Design review of the part built by this model. Coordinates are the model's own, in mm. A direction names the side the tool comes from. Coordinates: 2 decimals unless noted, no trailing zeros. Loops run counter-clockwise (first coordinate to the right, second up) from the corner with the lowest first, then second, coordinate; pieces in that order, holes last. Notation, with made-up numbers: M -2.5,56 L 27.5,56 A32 cw 27.5,89 Z; hole C -35.75,58.25 d4. An arc over 180 degrees is marked long. Answer as CSV lines item,"result". Start each with the question number.
from build123d import *

# Parameters (mm, degrees)
ESQUISSE1_W             = 55
ESQUISSE1_H             = 20
BOSS_EXTRU_1_DEPTH      = 10
ESQUISSE2_R             = 2
ENL_V_MAT_EXTRU_1_DEPTH = 20
ESQUISSE3_R             = 1.5
ESQUISSE3_W             = 23
ESQUISSE3_H             = 13
ENL_V_MAT_EXTRU_2_DEPTH = 20
BOSS_EXTRU_2_DEPTH      = 15
ENL_V_MAT_EXTRU_3_DEPTH = 15
ESQUISSE7_W             = 35
ESQUISSE7_H             = 20
ENL_V_MAT_EXTRU_4_DEPTH = 5


with BuildPart() as part:
    # Esquisse1 → Boss.-Extru.1 (new body)
    with BuildSketch(Plane.XY):
        with Locations((-0.833333333, -1.666666667)):
            Rectangle(ESQUISSE1_W, ESQUISSE1_H)
    extrude(amount=BOSS_EXTRU_1_DEPTH)

    # Esquisse2 → Enlèv. mat.-Extru.1 (cut)
    with BuildSketch(Plane(origin=(0, 8.333333333, 0), x_dir=(1, 0, 0), z_dir=(0, 1, 0))):
        with Locations(Location((-23.333333333, -5.548124667, 0), (0, 0, 270))):
            Circle(ESQUISSE2_R)
        with Locations(Location((-13.333333333, -5.548124667, 0), (0, 0, 270))):
            Circle(ESQUISSE2_R)
    extrude(amount=-ENL_V_MAT_EXTRU_1_DEPTH, mode=Mode.SUBTRACT)

    # Esquisse3 → Enlèv. mat.-Extru.2 (cut)
    with BuildSketch(Plane.XY.offset(10)):
        with Locations((24.166666667, -1.666666667)):
            Circle(ESQUISSE3_R)
        with Locations((-3.833333333, -1.666666667)):
            Circle(ESQUISSE3_R)
        with Locations((10.166666667, -1.666666667)):
            Rectangle(ESQUISSE3_W, ESQUISSE3_H)
    extrude(amount=-ENL_V_MAT_EXTRU_2_DEPTH, mode=Mode.SUBTRACT)

    # Esquisse5 → Boss.-Extru.2 (add)
    with BuildSketch(Plane(origin=(0, 0, 0), x_dir=(-1, 0, 0), z_dir=(0, 0, -1))):
        Polygon((28.333333333, -11.666666667), (28.333333333, 8.333333333), (8.333333333, 8.333333333), (8.333333333, -10.066666667), align=None)
    extrude(amount=BOSS_EXTRU_2_DEPTH)

    # Esquisse6 → Enlèv. mat.-Extru.3 (cut)
    with BuildSketch(Plane(origin=(0, 0, 0), x_dir=(-1, 0, 0), z_dir=(0, 0, -1))):
        Polygon((8.333333333, -10.066666667), (8.333333333, -11.666666667), (28.333333333, -11.666666667), align=None)
    extrude(amount=-ENL_V_MAT_EXTRU_3_DEPTH, mode=Mode.SUBTRACT)

    # Esquisse7 → Enlèv. mat.-Extru.4 (cut)
    with BuildSketch(Plane(origin=(0, 0, 0), x_dir=(-1, 0, 0), z_dir=(0, 0, -1))):
        with Locations((-9.166666667, -1.666666667)):
            Rectangle(ESQUISSE7_W, ESQUISSE7_H)
    extrude(amount=-ENL_V_MAT_EXTRU_4_DEPTH, mode=Mode.SUBTRACT)


solid = part.part
Item 1: For pin 1 (4 mm diameter, centred on x = 24.17, y = -1.67, fed in from -Z), flat-tipped, find the tip position at first contact; note if it passes through.
Item 2: Add section C-C (z = -10.5). Give the boundary of the cut face in (x, y).
Item 3: For faces 1 (the face through (-18.193, -10.855, -2.325)), 2 (the face through (10, 4.833, 8)), 3 (the face through (-8.333, -1, -5)), list the 3-axis set-ups (+Z, -Z, +X, -X, +Y, -Y) from which the entire face can be reached by the end or side of a thin tool; tool diameter is ignored.
Item 4: Add section A-A (y = 3.5). Give the boundary of the cut face in (x, z), plus the area to 3 significant figures.
Item 5: Add section D-D (x = -19). Give the boundary of the cut face in (y, z).
Item 6: For line 1 along X through (y, z) = (0.5, 9.25); line 2 along X through (y, z) = (1.75, 6.5); line 3 along Z through (x, y) = (22.5, 0.75), list the stretches that pass through material, from the lowest coordinate up. Write a range as from..to.
Item 7: Mouldability with a two-part tool opening along X and no side actions: class faces 4 (the face through (10, -8.167, 8)), 5 (the face through (-13, 8.333, 0)), 6 (the face through (-28.333, -2, -2)) as released by +X, released by -X, zero draft, split by the parting line, or undercut.
Item 8: Add section B-B (x = 1.5). Give the boundary of the cut face in (y, z).
Response:
1,pin 1,"z = 5"
2,outline,"M -28.33,-11.67 L -8.33,-10.07 L -8.33,8.33 L -28.33,8.33 Z"
3,face 1,"+Z, -Z, -Y"
3,face 2,"+Z, -Z"
3,face 3,"-Z, +X, +Y, -Y"
4,outline,"M -28.33,-15 L -8.33,-15 L -8.33,5 L -1.33,5 L -1.33,10 L -28.33,10 Z; M 21.67,5 L 26.67,5 L 26.67,10 L 21.67,10 Z; hole C -23.33,5.55 d4; hole C -13.33,5.55 d4"
4,area,"535 mm²"
5,outline,"M -10.92,-15 L 8.33,-15 L 8.33,10 L -10.92,10 Z"
6,line 1,"-28.33..-1.33, 21.67..26.67"
6,line 2,"-28.33..-25.09, -21.57..-15.09, -11.57..-1.33, 21.67..26.67"
6,line 3,"5..10"
7,face 4,"undercut"
7,face 5,"zero draft"
7,face 6,"released by -X"
8,outline,"M -11.67,5 L -8.17,5 L -8.17,10 L -11.67,10 Z; M 4.83,5 L 8.33,5 L 8.33,10 L 4.83,10 Z"
